Part model, mm, in its own coordinate system. A direction names the side the tool comes from. Round coordinates to 2 decimals unless told otherwise and drop trailing zeros. Put each result on its own line as item: value.
from build123d import *

# Parameters (mm, degrees)
BOSS_EXTRUDE1_DEPTH = 5


with BuildPart() as part:
    # Sketch2 → Boss-Extrude1 (new, symmetric)
    with BuildSketch(Plane(origin=(0, 0, 0), x_dir=(1, 0, 0), z_dir=(0, 1, 0))):
        with BuildLine():
            Line((-26.256733318, -4.621811883), (26.256733318, 4.621811883))
            add(Edge.make_bspline(
                [(26.256733318, 4.621811883), (26.184213815, 15.085916031), (31.39165321, 29.814258677), (31.49706253, 51.001483219), (32.310967161, 61.220682563), (33.852524137, 66.913865214)],
                knots=[0, 0, 0, 0, 0.494424997, 0.733347689, 1, 1, 1, 1], degree=3))
            Line((33.852524137, 66.913865214), (40.738782221, 92.345766637))
            Line((40.738782221, 92.345766637), (43.646124542, 106.427209936))
            Line((43.646124542, 106.427209936), (44.883071586, 123.411989276))
            add(Edge.make_bspline(
                [(44.883071586, 123.411989276), (45.165968858, 127.296511075), (39.51243958, 133.247924763), (34.10170013, 127.000274405), (33.459732834, 123.660322727)],
                knots=[0, 0, 0, 0, 0.483944054, 1, 1, 1, 1], degree=3))
            Line((33.459732834, 123.660322727), (30.874052834, 110.20785199))
            add(Edge.make_bspline(
                [(30.874052834, 110.20785199), (30.441188575, 107.955796914), (30.382492539, 103.306549634), (26.469197062, 99.749533646), (26.401505216, 97.069243348)],
                knots=[0, 0, 0, 0, 0.456305085, 1, 1, 1, 1], degree=3))
            Line((26.401505216, 97.069243348), (24.112480314, 86.815627265))
            add(Edge.make_bspline(
                [(19.297009656, 85.594758963), (19.243310028, 84.436078608), (19.094221788, 83.779551656), (20.94092685, 83.84883977), (22.432820011, 84.791228368), (23.934643349, 86.019012094), (24.112480314, 86.815627265)],
                knots=[0, 0, 0, 0, 0.237088594, 0.343164698, 0.637099032, 1, 1, 1, 1], degree=3))
            Line((19.297009656, 85.594758963), (20.36986935, 108.743922061))
            add(Edge.make_bspline(
                [(20.36986935, 108.743922061), (18.251278635, 120.569230524), (20.184141466, 132.474697955)],
                knots=[0, 0, 0, 1, 1, 1], degree=2))
            Line((20.184141466, 132.474697955), (21.422956498, 148.01825596))
            add(Edge.make_bspline(
                [(7.886453521, 151.373444104), (8.061393397, 154.365422898), (14.846563419, 158.831947186), (21.951965108, 154.65578924), (21.422956498, 148.01825596)],
                knots=[0, 0, 0, 0, 0.394994292, 1, 1, 1, 1], degree=3))
            Line((7.886453521, 151.373444104), (6.902699472, 134.548399342))
            Line((6.902699472, 134.548399342), (3.833351323, 110.20785199))
            Line((3.833351323, 110.20785199), (3.066920681, 95.274901286))
            add(Edge.make_bspline(
                [(-0.02159186, 96.268060872), (0.027684192, 94.213368932), (0.698982676, 92.143081029), (2.980886645, 93.598634774), (3.066920681, 95.274901286)],
                knots=[0, 0, 0, 0, 0.545550965, 1, 1, 1, 1], degree=3))
            Line((-0.02159186, 96.268060872), (-0.548678979, 118.246316572))
            add(Edge.make_bspline(
                [(-0.548678979, 145.251149648), (-0.915294678, 138.529010173), (-3.210810949, 131.270798089), (0.756296252, 121.816903372), (-0.548678979, 118.246316572)],
                knots=[0, 0, 0, 0, 0.597212586, 1, 1, 1, 1], degree=3))
            Line((-0.548678979, 145.251149648), (-0.02159186, 154.915637957))
            add(Edge.make_bspline(
                [(-14.082777353, 163.613875502), (-13.206305071, 169.295741696), (1.271215934, 168.230121804), (0.295217837, 160.724551686), (-0.02159186, 154.915637957)],
                knots=[0, 0, 0, 0, 0.553573038, 1, 1, 1, 1], degree=3))
            Line((-14.082777353, 163.613875502), (-14.082777353, 157.668307031))
            Line((-14.082777353, 157.668307031), (-15.437192564, 146.056382878))
            add(Edge.make_bspline(
                [(-18.807351222, 118.246316572), (-18.982381461, 121.2419879), (-18.455286153, 126.104488932), (-15.165218042, 135.219180874), (-15.95219543, 141.641064615), (-15.437192564, 146.056382878)],
                knots=[0, 0, 0, 0, 0.292833424, 0.552751335, 1, 1, 1, 1], degree=3))
            Line((-18.807351222, 118.246316572), (-17.5232119, 96.268060872))
            add(Edge.make_bspline(
                [(-17.5232119, 96.268060872), (-17.478594365, 95.504424428), (-17.663345633, 93.471140535), (-20.69353647, 90.530305698), (-21.741686411, 96.30347421), (-22.907109211, 102.276516742), (-22.86389916, 101.686280236)],
                knots=[0, 0, 0, 0, 0.194417097, 0.332418866, 0.645495928, 1, 1, 1, 1], degree=3))
            Line((-22.86389916, 101.686280236), (-23.90977525, 115.972638208))
            Line((-23.90977525, 115.972638208), (-27.993649806, 139.977396961))
            Line((-27.993649806, 139.977396961), (-28.550247244, 151.373444104))
            add(Edge.make_bspline(
                [(-42.440153209, 148.603290137), (-42.440153209, 156.79216036), (-37.316684629, 164.65280226), (-28.960959781, 159.782572709), (-28.550247244, 151.373444104)],
                knots=[0, 0, 0, 0, 0.53295506, 1, 1, 1, 1], degree=3))
            Line((-42.440153209, 148.603290137), (-42.440153209, 136.189708956))
            add(Edge.make_bspline(
                [(-41.668742375, 113.346816451), (-42.19497911, 116.743472309), (-42.99597028, 120.794670458), (-40.892054429, 129.161378833), (-42.440153209, 132.975454736), (-42.440153209, 136.189708956)],
                knots=[0, 0, 0, 0, 0.356023336, 0.669759724, 1, 1, 1, 1], degree=3))
            Line((-41.668742375, 113.346816451), (-39.481532119, 99.229214921))
            add(Edge.make_bspline(
                [(-39.481532119, 78.865982655), (-40.911565275, 83.601148767), (-39.535583433, 90.33311796), (-39.159502682, 97.150638681), (-39.481532119, 99.229214921)],
                knots=[0, 0, 0, 0, 0.695290511, 1, 1, 1, 1], degree=3))
            Line((-39.481532119, 78.865982655), (-39.481532119, 58.869061477))
            ThreePointArc((-39.481532119, 58.869061477), (-41.025725344, 56.493083351), (-43.824049084, 56.939389322))
            Line((-43.824049084, 56.939389322), (-51.36854474, 63.752158858))
            add(Edge.make_bspline(
                [(-58.832024896, 78.898041634), (-58.300951882, 75.958851634), (-56.370745123, 70.436918613), (-53.409290505, 65.594976618), (-51.36854474, 63.752158858)],
                knots=[0, 0, 0, 0, 0.533943101, 1, 1, 1, 1], degree=3))
            add(Edge.make_bspline(
                [(-58.832024896, 78.898041634), (-59.478052008, 82.473437818), (-63.45603922, 88.190679665), (-68.86425409, 93.338806019), (-71.187669739, 97.817450241), (-73.65768789, 98.799246852), (-78.090300121, 96.062640584), (-83.851775402, 94.152494508), (-80.98007287, 90.259003836)],
                knots=[0, 0, 0, 0, 0.267502676, 0.557706983, 0.582680153, 0.669254855, 0.724556218, 1, 1, 1, 1], degree=3))
            add(Edge.make_bspline(
                [(-80.98007287, 90.259003836), (-75.738710871, 84.470000229), (-73.6189357, 76.77203837), (-70.391217911, 69.829235803)],
                knots=[0, 0, 0, 0, 1, 1, 1, 1], degree=3))
            add(Edge.make_bspline(
                [(-70.391217911, 69.829235803), (-66.692008689, 62.860526967), (-62.867029651, 52.543349529), (-60.086598326, 42.060405741), (-58.905467069, 39.24574179)],
                knots=[0, 0, 0, 0, 0.723669094, 1, 1, 1, 1], degree=3))
            add(Edge.make_bspline(
                [(-26.256733318, -4.621811883), (-28.60669032, 0.892454726), (-39.270850453, 4.868841767), (-44.850488779, 18.875590893), (-52.803189433, 28.816690746), (-57.345558393, 35.528442216), (-58.905467069, 39.24574179)],
                knots=[0, 0, 0, 0, 0.306364848, 0.556646261, 0.785775409, 1, 1, 1, 1], degree=3))
        make_face()
    extrude(amount=BOSS_EXTRUDE1_DEPTH, both=True)


solid = part.part
1. Pin check, flat tips, straight feed: P1, Ø3, axis at y = -2, z = -42.5, coming from the +X side; P2, Ø6, axis at y = 2.5, z = -72.5, coming from the -X side; P3, Ø1.8, axis at y = 0.5, z = -161.5, coming from the -X side. Stop position of each tip, or through.
A:
P1: stops at x = 31.45
P2: stops at x = -72.82
P3: stops at x = -38.38
2. Probe line 1 along X through (y, z) = (-2.5, -112); line 2 along X through (y, z) = (3.5, -108); line 3 along X through (y, z) = (4, -142). List the from-to ranges inside material, lowest first. Write a range as [from, to].
A:
line 1: x = [-41.46, -23.62], [-18.44, -0.4], [4.06, 19.86], [31.22, 44.05]
line 2: x = [-40.84, -23.33], [-18.21, -0.3], [3.72, 20.34], [30.53, 43.76]
line 3: x = [-42.44, -28.09], [-15.69, -0.81], [7.34, 20.94]
3. Two-plate mould, pull along Z, no slides. Class faces 4 (the flat face through (7.4, 0.07, -143.08)), 5 (the flat face through (-0.29, 0.07, -150.02)), 6 (the flat face through (44.256, 0.07, -114.801)): pulls with the +Z half, pulls with the -Z half, needs draft (parallel to the pull), parting line crosses it, or undercut.
A:
face 4: pulls with the -Z half
face 5: undercut
face 6: pulls with the +Z half
4. Tool access for faces 1 (the cylindrical face through (-40.99, 0.07, -56.51)), 2 (the flat face through (-14.75, 0.07, -151.94)), 3 (the flat face through (-40.59, 0.07, -106.39)): list every direction of +Z, -Z, +X, -X, +Y, -Y with a clear straight run to the whole face (end or side of a thin tool).
A:
face 1: +Y, -Y
face 2: -Z, +Y, -Y
face 3: -X, +Y, -Y
